Work out the finished part from the listing and answer in its coordinate system (mm). Round coordinates to 2 decimals unless told otherwise and drop trailing zeros. Write each loop counter-clockwise with the first axis right and the second up, starting at its lowest first coordinate (ties: lowest second). Pieces come first, ordered by that corner, then holes. Notation, with made-up numbers: (-2.5, -31) -> (14.5, -31) arc R33 ccw to (14.5, 7) -> close; hole circle Ø4 at (44, -3). An arc over 180 degrees is marked (long way). Answer as a JSON object with one key per item and string values. Group by question number.
Autodesk Inventor part; units mm, degrees
ref_plane "1_XY" through (1.5, 0, 0) normal (1, 0, 0) x (0, 0, -1)
ref_plane "1_YZ" through (1.5, 0, 0) normal (0, 0, -1) x (0, 1, 0)
ref_plane "1_ZX" through (1.5, 0, 0) normal (0, 1, 0) x (1, 0, 0)
sketch "Sketch_5" plane through (0, 0, 0) normal (0, 0, 1) x (1, 0, 0)
  line L0 (3, 0) -> (0, 0)
  line L1 (0, 3.425) -> (0, 3.1)
  arc A0 (0, 3.1) -> (0.1, 3) centre (0.1, 3.1) ccw
  line L2 (0.1, 3) -> (2.9, 3)
  arc A1 (2.9, 3) -> (3, 3.1) centre (2.9, 3.1) ccw
  line L3 (3, 3.1) -> (3, 3.425)
  arc A2 (3, 3.425) -> (2.95, 3.475) centre (2.95, 3.425) ccw
  line L4 (2.95, 3.475) -> (1.7806, 3.475)
  arc A3 (1.2194, 3.475) -> (1.7806, 3.475) centre (1.5, 4) ccw
  line L5 (1.2194, 3.475) -> (0.05, 3.475)
  arc A4 (0.05, 3.475) -> (0, 3.425) centre (0.05, 3.425) ccw
revolve "Revolution1" add sketch "Sketch_5" angle 360 about axis through (3, 0, 0) along (1, 0, 0)
ref_plane "1_XY" through (1.5, 0, 0) normal (1, 0, 0) x (0, 0, -1)
ref_plane "1_YZ" through (1.5, 0, 0) normal (0, 0, -1) x (0, 1, 0)
ref_plane "1_ZX" through (1.5, 0, 0) normal (0, 1, 0) x (1, 0, 0)
ref_plane "Dummy_XY" through (0, 0, 0) normal (1, 0, 0) x (0, 0, -1)
ref_plane "Dummy_YZ" through (0, 0, 0) normal (0, 0, -1) x (0, 1, 0)
ref_plane "Dummy_ZX" through (0, 0, 0) normal (0, 1, 0) x (1, 0, 0)
ref_plane "shield1_XY" through (0.4, 0, 0) normal (1, 0, 0) x (0, 0, -1)
ref_plane "shield1_YZ" through (0.4, 0, 0) normal (0, 0, -1) x (0, 1, 0)
ref_plane "shield1_ZX" through (0.4, 0, 0) normal (0, 1, 0) x (1, 0, 0)
ref_plane "shield2_XY" through (2.6, 0, 0) normal (-1, 0, 0) x (0, 0, -1)
ref_plane "shield2_YZ" through (2.6, 0, 0) normal (0, 0, -1) x (0, -1, 0)
ref_plane "shield2_ZX" through (2.6, 0, 0) normal (0, -1, 0) x (-1, 0, 0)
properties part number "LF-1060ZZ_ir" material "鋼、炭素鋼"
1) A cutting plane is placed at C-C on x = 0.3. Determine the outline of the cut face in (y, z) (3 decimals).
2) Each of these flat-tipped pins is pushed along its axis until it touches: P1, Ø1, axis at x = 1.5, z = -0.5, coming from the -Y side; P2, Ø1, axis at x = 2, y = 1, coming from the -Z side; P3, Ø2, axis at y = 0, z = 0.5, coming from the -X side. Where does it stop, or does it pass through?
3) A cutting plane is placed at A-A on z = 0. Determine the outline of the cut face in (x, y) (3 decimals), plus the area to 3 significant figures.
4) For a pull along Z with two mould halves and no side action, classify faces 1 (the face through (2, -3, 0)), 2 (the face through (0.627, -0.753, 3.392)) as released by +Z, released by -Z, zero draft, split by the parting line, or undercut.
5) Straight lines are drawn through the part: L1, parallel to Z at x = 0.9, y = 0 (3 decimals); L2, parallel to Z at x = 1.65, y = 0; L3, parallel to Y at x = 0.75, z = -0.75. For each, find the intervals that lie inside material, in ascending order.
Established:
{
 "1": {"outline": "circle Ø6.95 at (0, 0); hole circle Ø6 at (0, 0)"},
 "2": {"P1": "stops at y = -3.47", "P2": "stops at z = -3.44", "P3": "passes through"},
 "3": {"outline": "(0, -3.425) arc R0.05 ccw to (0.05, -3.475) -> (1.219, -3.475) arc R0.595 cw to (1.781, -3.475) -> (2.95, -3.475) arc R0.05 ccw to (3, -3.425) -> (3, -3.1) arc R0.1 ccw to (2.9, -3) -> (0.1, -3) arc R0.1 ccw to (0, -3.1) -> close; (0, 3.1) arc R0.1 ccw to (0.1, 3) -> (2.9, 3) arc R0.1 ccw to (3, 3.1) -> (3, 3.425) arc R0.05 ccw to (2.95, 3.475) -> (1.781, 3.475) arc R0.595 cw to (1.219, 3.475) -> (0.05, 3.475) arc R0.05 ccw to (0, 3.425) -> close", "area": "2.79 mm²"},
 "4": {"face 1": "undercut", "face 2": "split by the parting line"},
 "5": {"L1": "z = -3.475 to -3, 3 to 3.475", "L2": "z = -3.42 to -3, 3 to 3.42", "L3": "y = -3.39 to -2.9, 2.9 to 3.39"}
}
